```python
from build123d import *

# Parameters (mm, degrees)
SKETCH2_R           = 15
BOSS_EXTRUDE1_DEPTH = 8.39
SHELL1_T            = -3
SKETCH3_R           = 1.25
CUT_EXTRUDE1_DEPTH  = 5
SCALE1_SCALE        = 0.5


with BuildPart() as part:
    # Sketch2 → Boss-Extrude1 (new body)
    with BuildSketch(Plane.XY):
        Circle(SKETCH2_R)
    extrude(amount=BOSS_EXTRUDE1_DEPTH)

    # Shell1
    shell1_openings = [part.faces().sort_by_distance(p)[0] for p in [
        (0, 0, 8.39),
    ]]
    offset(amount=SHELL1_T, openings=shell1_openings, kind=Kind.INTERSECTION)

    # Sketch3 → Cut-Extrude1 (cut)
    with BuildSketch(Plane(origin=(0, 0, 0), x_dir=(-1, 0, 0), z_dir=(0, 0, -1))):
        with Locations((0, 10)):
            Circle(SKETCH3_R)
        with Locations((8.660254038, 5)):
            Circle(SKETCH3_R)
        with Locations((8.660254038, -5)):
            Circle(SKETCH3_R)
        with Locations((0, -10)):
            Circle(SKETCH3_R)
        with Locations((-8.660254038, -5)):
            Circle(SKETCH3_R)
        with Locations((-8.660254038, 5)):
            Circle(SKETCH3_R)
    extrude(amount=-CUT_EXTRUDE1_DEPTH, mode=Mode.SUBTRACT)


with BuildPart() as part_1:
    # Scale1: scaled about (0, 0, 3.190405366)
    add(part.part.scale(SCALE1_SCALE).moved(Location((0, 0, 1.595202683))))


solid = part_1.part
```
Part model, mm, in its own coordinate system. A direction names the side the tool comes from. Coordinates: 2 decimals unless noted, no trailing zeros. Order: outer loops, then holes, each group sorted by start corner. A loop starts at its lowest first (then second) coordinate and runs counter-clockwise, first axis right, second up. Notation, with made-up numbers: (35.25, -4.5) - (78.25, -4.5) arc R8 cw to (78.25, -0.5) - close; hole circle Ø1 at (22.5, -28). An arc over 180 degrees is marked (long way). Return JSON: item names as keys, results as strings. Group by question number.
Item 1: Cut at A-A (x = 0). List the corners of the cut face in (y, z) (3 decimals).
Item 2: Cut at B-B (y = 2.5). List the corners of the cut face in (x, z), plus the area to 3 significant figures.
Item 3: Which spindle directions (+Z, -Z, +X, -X, +Y, -Y) get a long thin tool onto all of the face, cutting with end or side? Do faces 5 (the face through (0, 0, 3.095)), 6 (the face through (-4.19, -3.11, 2.33)). Say none if no direction does.
Item 4: Pin check, flat tips, straight feed: pin 1 (2 mm diameter, centred on x = 4.33, y = -2.5, fed in from -Z); pin 2 (6 mm diameter, centred on x = 0.5, y = -1.5, fed in from +Z); pin 3 (1 mm diameter, centred on y = -1.5, z = 2.5, fed in from +X). Stop position of each tip, or through.
Item 5: Drill centre lines: probe 1 along Y at (x, z) = (0, 2.3) (3 decimals); probe 2 along Y at (x, z) = (0, 4.15); probe 3 along Z at (x, y) = (-1, 2.5). Where is each one in solid material? Low to high. Write a range as from..to.
Item 6: Cut at C-C (x = -5.5). List the corners of the cut face in (y, z).
Item 7: Cut at D-D (y = -0.75). List the corners of the cut face in (x, z), plus the area to 3 significant figures.
Item 8: Pull direction Y, two halves, no side cores. Call faces 1 (the face through (3.753, -2.739, 2.335)), 2 (the face through (3.753, 2.261, 2.335)), 3 (the face through (2, 6, 5.79)), 4 (the face through (-7.493, 0.33, 3.663)): pulls with the +Y half, pulls with the -Y half, needs draft (parallel to the pull), parting line crosses it, or undercut.
Check values:
{
 "1": {"outline": "(-7.5, 1.595) - (-5.625, 1.595) - (-5.625, 3.095) - (-6, 3.095) - (-6, 5.79) - (-7.5, 5.79) - close; (-4.375, 1.595) - (4.375, 1.595) - (4.375, 3.095) - (-4.375, 3.095) - close; (5.625, 1.595) - (7.5, 1.595) - (7.5, 5.79) - (6, 5.79) - (6, 3.095) - (5.625, 3.095) - close"},
 "2": {"outline": "(-7.07, 1.6) - (-4.96, 1.6) - (-4.96, 3.1) - (-5.45, 3.1) - (-5.45, 5.79) - (-7.07, 5.79) - close; (-3.71, 1.6) - (3.71, 1.6) - (3.71, 3.1) - (-3.71, 3.1) - close; (4.96, 1.6) - (7.07, 1.6) - (7.07, 5.79) - (5.45, 5.79) - (5.45, 3.1) - (4.96, 3.1) - close", "area": "26.2 mm2"},
 "3": {"face 5": "+Z", "face 6": "+Z, -Z"},
 "4": {"pin 1": "stops at z = 1.6", "pin 2": "stops at z = 3.1", "pin 3": "stops at x = 7.43"},
 "5": {"probe 1": "y = -7.5..-5.625, -4.375..4.375, 5.625..7.5", "probe 2": "y = -7.5..-6, 6..7.5", "probe 3": "z = 1.6..3.1"},
 "6": {"outline": "(-5.1, 1.6) - (5.1, 1.6) - (5.1, 5.79) - (2.4, 5.79) - (2.4, 3.1) - (-2.4, 3.1) - (-2.4, 5.79) - (-5.1, 5.79) - close"},
 "7": {"outline": "(-7.46, 1.6) - (7.46, 1.6) - (7.46, 5.79) - (5.95, 5.79) - (5.95, 3.1) - (-5.95, 3.1) - (-5.95, 5.79) - (-7.46, 5.79) - close", "area": "30.5 mm2"},
 "8": {"face 1": "undercut", "face 2": "undercut", "face 3": "needs draft", "face 4": "parting line crosses it"}
}
